Could you check a few things on this drawing? It's one solid part, dimensions in mm from its lowest x, y, z. Coordinates: 2 decimals unless noted, no trailing zeros. Loops run counter-clockwise (first coordinate to the right, second up) from the corner with the lowest first, then second, coordinate; pieces in that order, holes last.
1) Imagine slicing it at A-A on x = 26.5. Please give me the cut outline in (y, z).
2) Will these pins go through, and if not, where does the flat tip stop? P1, Ø1.6, axis at y = 56, z = 2, coming from the +X side; P2, Ø1.5, axis at x = 78.5, z = 2, coming from the -Y side; P3, Ø1.2, axis at y = 2, z = 1.5, coming from the -X side; P4, Ø3, axis at x = 53, y = 29.5, coming from the -Z side.
3) If I drill on line 1 along Y through (x, z) = (30, 1.1); line 2 along Y through (x, z) = (60, 2.4), over which ranges is the centre line in solid material (lowest first)?
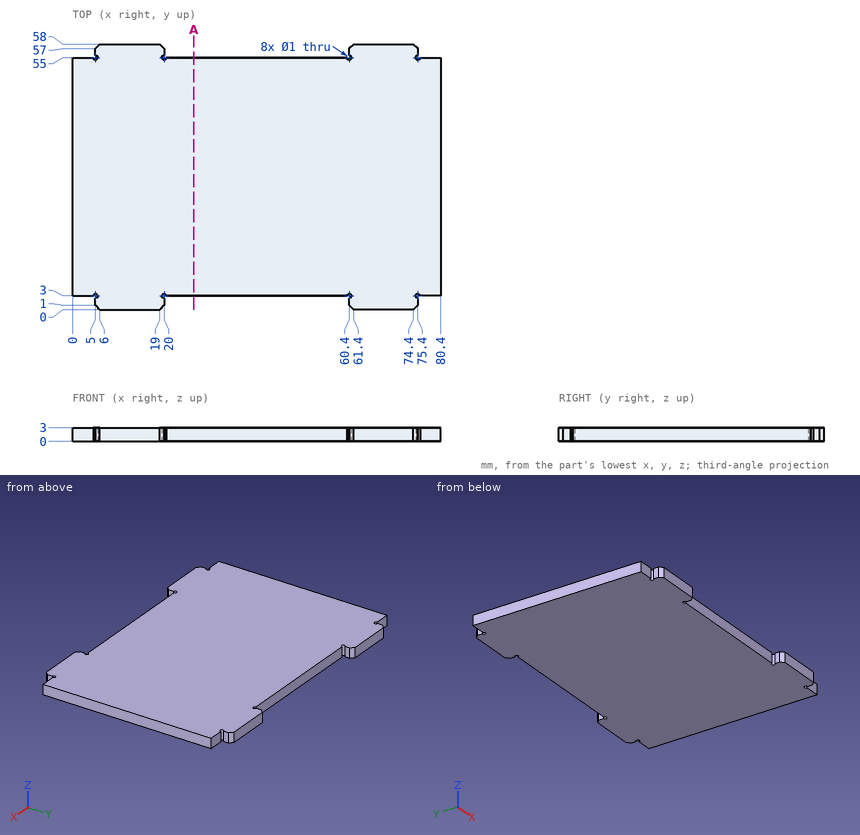
Filled in:
1. outline: (3, 0) - (55, 0) - (55, 3) - (3, 3) - close
2. P1: stops at x = 75.4
2. P2: stops at y = 3
2. P3: stops at x = 5
2. P4: stops at z = 0
3. line 1: y = 3 to 55
3. line 2: y = 3.3 to 54.7
